from build123d import *

# Parameters (mm, degrees)
SKETCH_1_R               = 2.8
EXTRUDE_1_DEPTH          = 35
SKETCH_2_W               = 0.5
SKETCH_2_H               = 5.450532248
CUT_EXTRUDE_1_DEPTH      = 12
CUT_EXTRUDE_2_DEPTH      = 10
CUT_EXTRUDE_2_DEPTH_BACK = 10
SKETCH_3_R               = 1
SKETCH_4_R               = 5.5
EXTRUDE_2_DEPTH          = 6
SKETCH_5_R               = 3.6
CUT_EXTRUDE_3_DEPTH      = 3
FILLET_1_R               = 5


with BuildPart() as part:
    # 草图1 → 凸台-拉伸1 (new body)
    with BuildSketch(Plane(origin=(0, 0, 0), x_dir=(0, 0, -1), z_dir=(1, 0, 0))):
        Circle(SKETCH_1_R)
    extrude(amount=EXTRUDE_1_DEPTH)

    # 草图2 → 切除-拉伸1 (cut)
    with BuildSketch(Plane.ZY):
        with Locations((0, 0.396255312)):
            Rectangle(SKETCH_2_W, SKETCH_2_H)
    extrude(amount=-CUT_EXTRUDE_1_DEPTH, mode=Mode.SUBTRACT)

    # 草图3 → 切除-拉伸2 (cut, two sides: drawn at the far end of the back side and taken through both)
    with BuildSketch(Plane(origin=(0, 0, 0.25), x_dir=(-1, 0, 0), z_dir=(0, 0, -1)).offset(-CUT_EXTRUDE_2_DEPTH_BACK)):
        with Locations(Location((-3, -0.005591523, 0), (0, 0, 270))):
            Circle(SKETCH_3_R)
    extrude(amount=CUT_EXTRUDE_2_DEPTH + CUT_EXTRUDE_2_DEPTH_BACK, mode=Mode.SUBTRACT)

    # 草图4 → 凸台-拉伸2 (add)
    with BuildSketch(Plane(origin=(35, 0, 0), x_dir=(0, 0, -1), z_dir=(1, 0, 0))):
        Circle(SKETCH_4_R)
    extrude(amount=-EXTRUDE_2_DEPTH)

    # 草图5 → 切除-拉伸3 (cut)
    with BuildSketch(Plane(origin=(35, 0, 0), x_dir=(0, 0, -1), z_dir=(1, 0, 0))):
        Circle(SKETCH_5_R)
    extrude(amount=-CUT_EXTRUDE_3_DEPTH, mode=Mode.SUBTRACT)

    # 圆角1
    # the kernel refuses this fillet: 5 mm, written as the material it adds along each edge
    with BuildSketch(Plane(origin=(29, 0, 0), x_dir=(0, 0, -1), z_dir=(0, 1, 0))) as fillet_1_piece_1:
        with BuildLine():
            CenterArc((7.8, 4.439594576), FILLET_1_R, 180, 62.612892497)
            Line((5.5, 0), (5.454, -0.088791892))
            ThreePointArc((5.454, -0.088791892), (4.15, -0.1), (2.8, -0.1))
            Line((2.8, -0.1), (2.7, 0))
            Line((2.7, 0), (2.7, 4.439594576))
            Line((2.7, 4.439594576), (2.8, 4.439594576))
        make_face()
    revolve(axis=Axis((29, 0, 0), (-1, 0, 0)))


solid = part.part
Build history of the part. All positions in model axes, mm. A direction names the side the tool comes from. Round coordinates to 2 decimals unless told otherwise and drop trailing zeros. Loops run counter-clockwise (first coordinate to the right, second up) from the corner with the lowest first, then second, coordinate; pieces in that order, holes last. Notation, with made-up numbers: (77.5, -10) -> (129.5, -10) arc R30 ccw to (129.5, 27) -> close; hole circle Ø5 at (55, 86.25). An arc over 180 degrees is marked (long way). Use CSV: the item, a comma, the result in double quotes. Start each with the question number.
Q1. Which spindle directions (+Z, -Z, +X, -X, +Y, -Y) get a long thin tool onto all of the face, cutting with end or side? Do faces 4 (the face through (32, 0, 0)), 5 (the face through (2.956, 0.993, 1.543)), 6 (the face through (6, 0, -0.25)). Say none if no direction does.
Q2. Drill centre lines: L1, parallel to Y at x = 33.6, z = 0; L2, parallel to Z at x = 6.5, y = 0; L3, parallel to X at y = -2.5, z = 0.5. Where is each one in solid material? Low to high.
Q3. Saw through at A-A on x = 3. Give the cut face in (y, z).
Q4. Flat gauge pins, fed straight in: pin 1 Ø1.5 at (x, y) = (15, 2) entering from -Z; pin 2 Ø1 at (x, z) = (29, 3) entering from +Y; pin 3 Ø4 at (x, y) = (8, 1) entering from +Z; pin 4 Ø1.8 at (x, y) = (3, -0.01) entering from -Z. Where does each tip first touch, or does it go through?
Q5. Saw through at C-C on x = 19. Give the cut face in (y, z).
Q6. Mould opens along Z. For faces 1 (the face through (12.11, 0.84, -2.67)), 2 (the face through (33.521, 1.081, -3.434)), 3 (the face through (35, -1, -4)) say: +Z half, -Z half, draft (parallel to the pull), parting line (faces both ways), or undercut.
Q7. Saw through at B-B on y = 0. Give the cut face in (x, z), and give its area (3 significant figures).
Solutions:
1,face 4,"+X"
1,face 5,"+Z, -Z"
1,face 6,"-X, +Y"
2,L1,"y = -5.5 to -3.6, 3.6 to 5.5"
2,L2,"z = -2.8 to -0.25, 0.25 to 2.8"
2,L3,"x = 0 to 32"
3,outline,"(-2.33, -0.25) -> (-2.33, 0.25) -> (-1.01, 0.25) -> (-1.01, 2.61) arc R2.8 ccw to (-1.01, -2.61) -> (-1.01, -0.25) -> close; (0.99, -2.62) arc R2.8 ccw to (2.79, -0.25) -> (0.99, -0.25) -> close; (0.99, 0.25) -> (2.79, 0.25) arc R2.8 ccw to (0.99, 2.62) -> close"
4,pin 1,"stops at z = -2.51"
4,pin 2,"stops at y = 4.9"
4,pin 3,"stops at z = 2.8"
4,pin 4,"passes through"
5,outline,"circle Ø5.6 at (0, 0)"
6,face 1,"parting line"
6,face 2,"undercut"
6,face 3,"draft"
7,outline,"(0, -2.8) -> (2, -2.8) -> (2, -0.25) -> (0, -0.25) -> close; (0, 0.25) -> (2, 0.25) -> (2, 2.8) -> (0, 2.8) -> close; (4, -2.8) -> (24.56, -2.8) arc R5 cw to (29, -5.5) -> (35, -5.5) -> (35, -3.6) -> (32, -3.6) -> (32, 3.6) -> (35, 3.6) -> (35, 5.5) -> (29, 5.5) arc R5 cw to (24.56, 2.8) -> (4, 2.8) -> (4, 0.25) -> (12, 0.25) -> (12, -0.25) -> (4, -0.25) -> close"
7,area,"197 mm^2"
